The listing builds one solid part. Answer for the finished solid, in the listing's coordinates (mm). Face numbers are marked on the shaded views. A direction names the side the tool comes from. Coordinates: 2 decimals unless noted, no trailing zeros. Loops run counter-clockwise (first coordinate to the right, second up) from the corner with the lowest first, then second, coordinate; pieces in that order, holes last. Notation, with made-up numbers: (45, 2) - (62, 2) arc R31 ccw to (62, 39) - close; hole circle Ø11 at (72, 7.25). An arc over 180 degrees is marked (long way). Write each question's results on one line, items separated by ' | '. Start each with the question number.
(1) Find section D-D on x = 32. Determine the outline of the cut face in (y, z).
(2) Find section B-B on x = 120. Determine the outline of the cut face in (y, z), then the cut area to 3 significant figures.
(3) For the marked faces 4 and 5, determine the directions among +Z, -Z, +X, -X, +Y, -Y from which every point of the face is accessible in a straight line to the end or side of a thin tool.
(4) Find section A-A on z = -9.75. Determine the outline of the cut face in (x, y).
(5) Given pin 1 Ø9.5 at (y, z) = (37.5, -14) entering from -X; pin 2 Ø8 at (x, z) = (29, -4) entering from -Y; pin 3 Ø6 at (y, z) = (2, -13.5) entering from -X, each flat-ended and moving along its own axis, determine where each tip first touches the part or whether it passes through.
(6) Consider line 1 (X direction, y = 330, z = -13.5); line 2 (Y direction, x = 142, z = -7.5); line 3 (X direction, y = 248.5, z = -15.5). Determine where each line is inside the solid, lowest interval first. Write a range as from..to.
(7) Find section C-C on y = 234. Determine the outline of the cut face in (x, z), then the cut area to 3 significant figures.
(8) Determine the mould class of the marked faces 1, 2 and 3 for opening direction Z: released by +Z, released by -Z, zero draft, split by the parting line, or undercut.
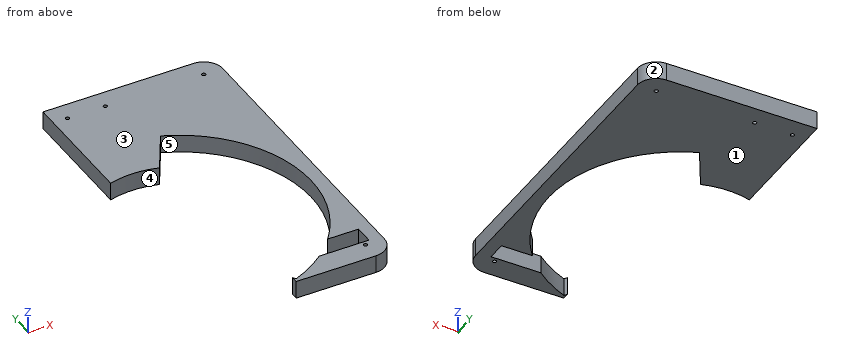
from build123d import *

# Parameters (mm, degrees)
PAD016_DEPTH    = 19
FILLET006_R     = 20
SKETCH023_R     = 2
POCKET014_DEPTH = 19.001
SKETCH026_R     = 2
POCKET016_DEPTH = 19.001
SKETCH047_W     = 56
SKETCH047_H     = 20
POCKET030_DEPTH = 19.001


with BuildPart() as part:
    # Sketch021 → Pad016 (new body)
    with BuildSketch(Plane.XY):
        with BuildLine():
            Line((200, 216.2), (200, 86.458082))
            ThreePointArc((251.554314, 85.993421), (225.811141, 89.996345), (200, 86.458082))
            Line((251.554314, 85.993421), (276.961524, 130))
            ThreePointArc((276.961524, -130), (365, 0), (276.961524, 130))
            Line((276.961524, -130), (275, -126.60254))
            Line((275, -126.60254), (275, -133.8))
            Line((275, -133.8), (379.498932, -133.8))
            Line((379.498932, -133.8), (379.498932, 216.2))
            Line((379.498932, 216.2), (200, 216.2))
        make_face()
    extrude(amount=PAD016_DEPTH)

    # Fillet006
    fillet006_edges = [part.edges().sort_by_distance(p)[0] for p in [
        (379.498932, 216.2, 9.5),
        (379.498932, -133.8, 9.5),
    ]]
    fillet(fillet006_edges, radius=FILLET006_R)

    # Sketch023 (on Face5 of Fillet006) → Pocket014 (cut, through all)
    with BuildSketch(Plane.XY.offset(19)):
        with Locations((215, 196.2)):
            Circle(SKETCH023_R)
    extrude(amount=-POCKET014_DEPTH, mode=Mode.SUBTRACT)

    # Sketch026 (on Face5 of Pocket014) → Pocket016 (cut, through all)
    with BuildSketch(Plane.XY.offset(19)):
        with Locations((254.998932, 196.2)):
            Circle(SKETCH026_R)
        with Locations((359.498932, 196.2)):
            Circle(SKETCH026_R)
        with Locations((359.498932, -113.8)):
            Circle(SKETCH026_R)
    extrude(amount=-POCKET016_DEPTH, mode=Mode.SUBTRACT)

    # Sketch047 (on Face2 of Pocket016) → Pocket030 (cut, through all)
    with BuildSketch(Plane(origin=(0, 0, 0), x_dir=(1, 0, 0), z_dir=(0, 0, -1))):
        with Locations((337.998932, 98.8)):
            Rectangle(SKETCH047_W, SKETCH047_H)
    extrude(amount=-POCKET030_DEPTH, mode=Mode.SUBTRACT)


with BuildPart() as part_1:
    # Body012 placement: moved
    add(part.part.moved(Location((0, 0, -9))))


with BuildPart() as part_2:
    # Clone placement: moved
    add(part_1.part.moved(Location((-200, 133.8, -10))))


solid = part_2.part
Values:
1) outline: (223.53, -19) - (350, -19) - (350, 0) - (223.53, 0) - close
2) outline: (0, -19) - (25, -19) - (25, 0) - (0, 0) - close; (236.63, -19) - (350, -19) - (350, 0) - (236.63, 0) - close | area: 2,630 mm²
3) face 4: +Z, -Z, -Y | face 5: +Z, -Z
4) outline: (0, 220.26) arc R90 cw to (51.55, 219.79) - (76.96, 263.8) arc R140 cw to (133.23, 45) - (166, 45) - (166, 25) - (113.11, 25) arc R140 cw to (76.96, 3.8) - (75, 7.2) - (75, 0) - (159.5, 0) arc R20 ccw to (179.5, 20) - (179.5, 330) arc R20 ccw to (159.5, 350) - (0, 350) - close; hole circle Ø4 at (15, 330); hole circle Ø4 at (55, 330); hole circle Ø4 at (159.5, 20); hole circle Ø4 at (159.5, 330)
5) pin 1: stops at x = 166 | pin 2: stops at y = 223.44 | pin 3: stops at x = 75
6) line 1: x = 0..13, 17..53, 57..157.5, 161.5..179.5 | line 2: y = 0..25, 45..56.92, 210.68..350 | line 3: x = 0..68.13, 105.27..179.5
7) outline: (0, -19) - (59.76, -19) - (59.76, 0) - (0, 0) - close; (122.78, -19) - (179.5, -19) - (179.5, 0) - (122.78, 0) - close | area: 2,210 mm²
8) face 1: released by -Z | face 2: zero draft | face 3: released by +Z
